Input: part model. Units: mm. Frame: model coordinates. Face numbers are marked on the shaded views. A direction names the side the tool comes from. Give positions to 0.01 mm unless a question says otherwise; leave off trailing zeros. Order: outer loops, then holes, each group sorted by start corner. A loop starts at its lowest first (then second) coordinate and runs counter-clockwise, first axis right, second up. Notation, with made-up numbers: (89.5, -8) - (97.5, -8) arc R29 cw to (97.5, 28) - close; hole circle Ø6 at (41, 6). An arc over 180 degrees is marked (long way). Answer in a Markdown table with one row per item. Add a question column.
1. Contact query for flat-ended pins moving along their axis: pin 1 (19 mm diameter, centred on x = -28.5, z = 58.5, fed in from +Y); pin 2 (13.5 mm diameter, centred on x = 85.5, z = 63, fed in from +Y); pin 3 (25 mm diameter, centred on x = -31.5, y = -6, fed in from +Z). Output: stop coordinate, or through.
2. Access query for the marked faces 5, 6 and 7. Directions: +Z, -Z, +X, -X, +Y, -Y. A direction counts if a zero-diameter tool reaches every point of the face in a straight line with its end or side. Return the directions, or none.
3. Ray query, line 1 (Y direction, x = 30, z = 66); line 2 (Z direction, x = 21.5, y = 33); line 3 (Z direction, x = -9, y = 22.5). Return the intervals inside material, ascending. Write a range as [from, to].
4. Section query B-B on z = 30. Count the separate pieces of the cut face and the enclosed holes in it, and give its area (3 significant figures).
5. Section query D-D on x = -17.5. Return loops of the section in (y, z).
6. Section query A-A on x = 30. Return loops of the section in (y, z), and give its area (3 significant figures).
7. Mould query, pull axis X, two halves, no side actions, for the marked faces 1, 2, 3 and 4. Classes: released by +X, released by -X, zero draft, split by the parting line, or undercut.
8. Section query C-C on y = 23.5. Return loops of the section in (x, z).
```python
from build123d import *

# Parameters (mm, degrees)
BOSS_EXTRUDE1_DEPTH = 40
BOSS_EXTRUDE2_DEPTH = 30
SKETCH3_R           = 20
BOSS_EXTRUDE3_DEPTH = 20
SKETCH4_R           = 10
CUT_EXTRUDE1_DEPTH  = 185
SKETCH5_R           = 5
CUT_EXTRUDE2_DEPTH  = 185
SKETCH6_R           = 5
CUT_EXTRUDE3_DEPTH  = 20
CUT_EXTRUDE4_DEPTH  = 20
CUT_EXTRUDE5_DEPTH  = 20
CUT_EXTRUDE7_DEPTH  = 10


with BuildPart() as part:
    # Sketch1 → Boss-Extrude1 (new body)
    with BuildSketch(Plane.XY):
        Polygon((0, 40.88699749), (-20, 40.88699749), (-20, 30.88699749), (-50, 10.88699749), (-50, -29.11300251), (-20, -49.11300251), (-20, -59.11300251), (0, -59.11300251), (0, -54.11300251), (60, -54.11300251), (60, -59.11300251), (80, -59.11300251), (80, -49.11300251), (110, -29.11300251), (110, 10.88699749), (80, 30.88699749), (80, 40.88699749), (60, 40.88699749), (60, 35.88699749), (0, 35.88699749), align=None)
    extrude(amount=BOSS_EXTRUDE1_DEPTH)

    # Sketch2 → Boss-Extrude2 (add)
    with BuildSketch(Plane.XY.offset(40)):
        with BuildLine():
            Line((0, 30.88699749), (15, 30.88699749))
            Line((15, 30.88699749), (15, 20.88699749))
            Line((15, 20.88699749), (45, 20.88699749))
            Line((45, 20.88699749), (45, 30.88699749))
            Line((45, 30.88699749), (60, 30.88699749))
            ThreePointArc((60, 30.88699749), (100, -9.11300251), (60, -49.11300251))
            Line((60, -49.11300251), (45, -49.11300251))
            Line((45, -49.11300251), (45, -39.11300251))
            Line((45, -39.11300251), (15, -39.11300251))
            Line((15, -39.11300251), (15, -49.11300251))
            Line((15, -49.11300251), (0, -49.11300251))
            ThreePointArc((0, -49.11300251), (-40, -9.11300251), (0, 30.88699749))
        make_face()
    extrude(amount=BOSS_EXTRUDE2_DEPTH)

    # Sketch3 → Boss-Extrude3 (add)
    with BuildSketch(Plane.XY.offset(70)):
        with Locations((30, -9.11300251)):
            Circle(SKETCH3_R)
    extrude(amount=BOSS_EXTRUDE3_DEPTH)

    # Sketch4 → Cut-Extrude1 (cut)
    with BuildSketch(Plane.XY.offset(90)):
        with Locations((30, -9.11300251)):
            Circle(SKETCH4_R)
    extrude(amount=-CUT_EXTRUDE1_DEPTH, mode=Mode.SUBTRACT)

    # Sketch5 → Cut-Extrude2 (cut)
    with BuildSketch(Plane.XY.offset(70)):
        with Locations((-20, -9.11300251)):
            Circle(SKETCH5_R)
        with Locations((80, -9.11300251)):
            Circle(SKETCH5_R)
    extrude(amount=-CUT_EXTRUDE2_DEPTH, mode=Mode.SUBTRACT)

    # Sketch6 → Cut-Extrude3 (cut)
    with BuildSketch(Plane.XY.offset(70)):
        with BuildLine():
            ThreePointArc((-20, -24.11300251), (-5, -9.11300251), (-20, 5.88699749))
            Line((-20, 5.88699749), (-37.080992435, 5.88699749))
            ThreePointArc((-37.080992435, 5.88699749), (-40, -9.11300251), (-37.080992435, -24.11300251))
            Line((-37.080992435, -24.11300251), (-20, -24.11300251))
        make_face()
        with Locations((-20, -9.11300251)):
            Circle(SKETCH6_R, mode=Mode.SUBTRACT)
        with BuildLine():
            Line((97.080992435, 5.88699749), (80, 5.88699749))
            ThreePointArc((80, 5.88699749), (65, -9.11300251), (80, -24.11300251))
            Line((80, -24.11300251), (97.080992435, -24.11300251))
            ThreePointArc((97.080992435, -24.11300251), (100, -9.11300251), (97.080992435, 5.88699749))
        make_face()
        with Locations((80, -9.11300251)):
            Circle(SKETCH6_R, mode=Mode.SUBTRACT)
    extrude(amount=-CUT_EXTRUDE3_DEPTH, mode=Mode.SUBTRACT)

    # Sketch7 → Cut-Extrude4 (cut)
    with BuildSketch(Plane.XY.offset(40)):
        Polygon((0, 35.88699749), (0, 30.88699749), (15, 30.88699749), (15, 20.88699749), (45, 20.88699749), (45, 30.88699749), (60, 30.88699749), (60, 35.88699749), align=None)
    extrude(amount=-CUT_EXTRUDE4_DEPTH, mode=Mode.SUBTRACT)

    # Sketch8 → Cut-Extrude5 (cut)
    with BuildSketch(Plane.XY.offset(40)):
        Polygon((0, -54.11300251), (0, -49.11300251), (15, -49.11300251), (15, -39.11300251), (45, -39.11300251), (45, -49.11300251), (60, -49.11300251), (60, -54.11300251), align=None)
    extrude(amount=-CUT_EXTRUDE5_DEPTH, mode=Mode.SUBTRACT)

    # Sketch9 → Cut-Extrude7 (cut)
    with BuildSketch(Plane(origin=(0, 0, 0), x_dir=(-1, 0, 0), z_dir=(0, 0, -1))):
        Polygon((-99.5, 17.88699749), (39.5, 17.88699749), (50, 10.88699749), (50, -29.11300251), (39.5, -36.11300251), (-99.5, -36.11300251), (-110, -29.11300251), (-110, 10.88699749), align=None)
    extrude(amount=-CUT_EXTRUDE7_DEPTH, mode=Mode.SUBTRACT)


solid = part.part
```
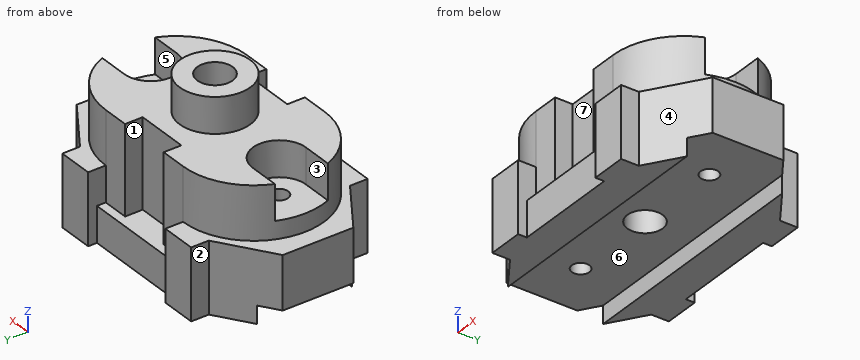
Answer:
| question | item | result |
|---|---|---|
| 1 | pin 1 | stops at y = 26.09 |
| 1 | pin 2 | stops at y = 26.22 |
| 1 | pin 3 | stops at z = 70 |
| 2 | face 5 | +Z, +X |
| 2 | face 6 | -Z, +X, -X |
| 2 | face 7 | +Z, -Y |
| 3 | line 1 | y = [-39.11, -19.11], [0.89, 20.89] |
| 3 | line 2 | z = [0, 20] |
| 3 | line 3 | z = [0, 70] |
| 4 | separate pieces | 1 |
| 4 | enclosed holes | 3 |
| 4 | area | 11,300 mm² |
| 5 | outline | (-59.11, 0) - (-36.11, 0) - (-36.11, 10) - (-13.44, 10) - (-13.44, 50) - (-23.9, 50) - (-23.9, 70) - (-45.08, 70) - (-45.08, 40) - (-59.11, 40) - close; (-4.78, 10) - (17.89, 10) - (17.89, 0) - (40.89, 0) - (40.89, 40) - (26.86, 40) - (26.86, 70) - (5.68, 70) - (5.68, 50) - (-4.78, 50) - close |
| 6 | outline | (-54.11, 0) - (-36.11, 0) - (-36.11, 10) - (-19.11, 10) - (-19.11, 90) - (-29.11, 90) - (-29.11, 70) - (-39.11, 70) - (-39.11, 20) - (-54.11, 20) - close; (0.89, 10) - (17.89, 10) - (17.89, 0) - (35.89, 0) - (35.89, 20) - (20.89, 20) - (20.89, 70) - (10.89, 70) - (10.89, 90) - (0.89, 90) - close |
| 6 | area | 3,460 mm² |
| 7 | face 1 | undercut |
| 7 | face 2 | released by -X |
| 7 | face 3 | zero draft |
| 7 | face 4 | released by +X |
| 8 | outline | (-31.08, 0) - (91.08, 0) - (91.08, 40) - (83.16, 40) - (83.16, 70) - (45, 70) - (45, 20) - (15, 20) - (15, 70) - (-23.16, 70) - (-23.16, 40) - (-31.08, 40) - close |
